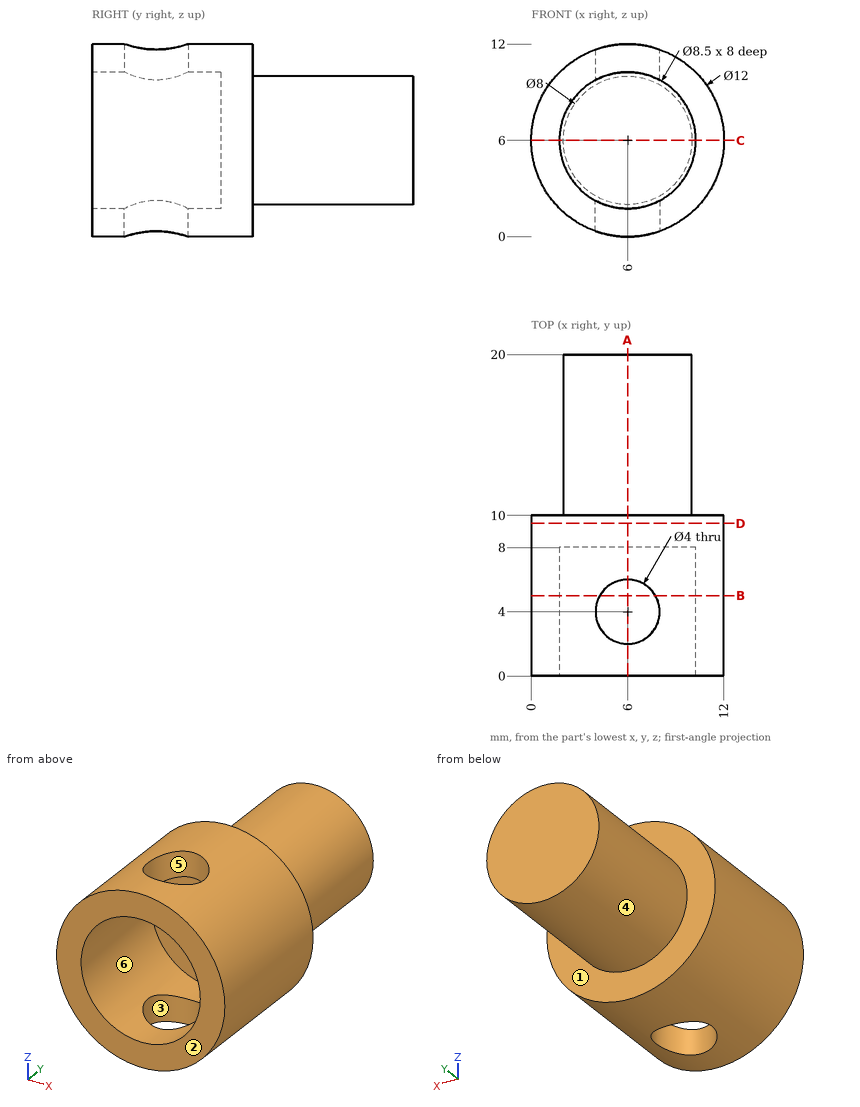
Job drawing, mm, ordinate dimensions from the low corner. One solid piece. A direction names the side the tool comes from. Round coordinates to 2 decimals unless told otherwise and drop trailing zeros. Loops run counter-clockwise (first coordinate to the right, second up) from the corner with the lowest first, then second, coordinate; pieces in that order, holes last. Notation, with made-up numbers: M 44,13.25 L 100,13.25 A8 cw 100,28.25 Z; hole C 60,-2 d11. An arc over 180 degrees is marked long. One line per question, with ' | ' between items. Start each with the question number.
Item 1: Pin check, flat tips, straight feed: pin 1 Ø2 at (y, z) = (12.5, 7.5) entering from +X; pin 2 Ø4 at (x, z) = (6, 7.5) entering from -Y; pin 3 Ø5 at (x, z) = (9.5, 1.5) entering from +Y; pin 4 Ø6 at (x, y) = (7, 14.5) entering from -Z. Stop position of each tip, or through.
Item 2: Two-plate mould, pull along Y, no slides. Class the marked faces 1, 2 and 3: pulls with the +Y half, pulls with the -Y half, needs draft (parallel to the pull), parting line crosses it, or undercut.
Item 3: Cut at D-D, the plane y = 9.5. Write the cut outline in (x, z).
Item 4: Which spindle directions (+Z, -Z, +X, -X, +Y, -Y) get a long thin tool onto all of the face, cutting with end or side? Do the marked faces 4, 5 and 6. Say none if no direction does.
Item 5: Wall check: line 1 (Y direction, x = 6, z = 0.7); line 2 (Y direction, x = 5, z = 4.5); line 3 (Y direction, x = 11, z = 7). Give the ranges that are in metal, low to high.
Item 6: Cut at C-C, the plane z = 6. Write the cut outline in (x, y).
Item 7: Cut at A-A, the plane x = 6. Write the cut outline in (y, z).
Item 8: Cut at B-B, the plane y = 5. Write the cut outline in (x, z).
Responses:
1) pin 1: stops at x = 9.97 | pin 2: stops at y = 8 | pin 3: stops at y = 20 | pin 4: stops at z = 2
2) face 1: pulls with the +Y half | face 2: pulls with the -Y half | face 3: undercut
3) outline: C 6,6 d12
4) face 4: +Y | face 5: +Z, -Z | face 6: -Y
5) line 1: y = 0 to 2, 6 to 10 | line 2: y = 8 to 20 | line 3: y = 0 to 10
6) outline: M 0,0 L 1.75,0 L 1.75,8 L 10.25,8 L 10.25,0 L 12,0 L 12,10 L 10,10 L 10,20 L 2,20 L 2,10 L 0,10 Z
7) outline: M 0,0 L 2,0 L 2,1.75 L 0,1.75 Z; M 0,10.25 L 2,10.25 L 2,12 L 0,12 Z; M 6,0 L 10,0 L 10,2 L 20,2 L 20,10 L 10,10 L 10,12 L 6,12 L 6,10.25 L 8,10.25 L 8,1.75 L 6,1.75 Z
8) outline: M 4.27,0.26 L 4.27,2.12 A4.25 cw 4.27,9.88 L 4.27,11.74 A6 ccw Z; M 7.73,0.26 A6 ccw 7.73,11.74 L 7.73,9.88 A4.25 cw 7.73,2.12 Z
